Read the model definition and answer for the solid it produces. Units are mm, in the model's axes. Face numbers are marked on the shaded views. A direction names the side the tool comes from. Coordinates: 2 decimals unless noted, no trailing zeros. Order: outer loops, then holes, each group sorted by start corner. A loop starts at its lowest first (then second) coordinate and runs counter-clockwise, first axis right, second up. Notation, with made-up numbers: (80, -3) -> (106, -3) arc R14 ccw to (106, 18) -> close; hole circle Ø8 at (74, 9.5). An arc over 180 degrees is marked (long way). Use CSV: the item, a comma, the result in double quotes.
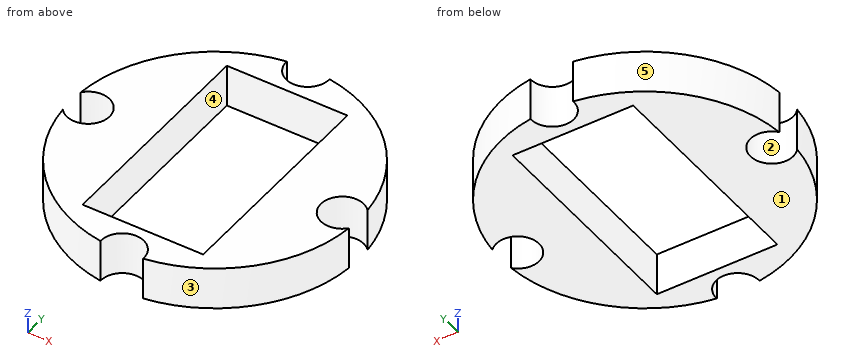
Autodesk Inventor part; units mm, degrees
ref_plane "YZ Plane" through (0, 0, 0) normal (1, 0, 0) x (0, 1, 0)
ref_plane "XZ Plane" through (0, 0, 0) normal (0, 1, 0) x (-1, 0, 0)
ref_plane "XY Plane" through (0, 0, 0) normal (0, 0, 1) x (1, 0, 0)
sketch "Sketch3" plane through (0, 0, 0) normal (0, 0, 1) x (1, 0, 0)
  line L0 (-15.9263, -16.7) -> (16.0737, -16.7)
  line L1 (16.7744, -15.9999) -> (16.6729, 15.9999)
  line L2 (15.9735, 16.7) -> (-16.0265, 16.7)
  line L3 (-16.7272, 15.9999) -> (-16.6257, -15.9999)
  line L4 (-16.0265, 16.7) -> (-16.7272, 15.9999)
  line L5 (15.9735, 16.7) -> (16.6729, 15.9999)
  line L6 (16.7744, -15.9999) -> (16.0737, -16.7)
  line L7 (-16.6257, -15.9999) -> (-15.9263, -16.7)
  line L8 (-5.7625, -10.525) -> (5.7625, -10.525)
  line L9 (5.7625, -10.525) -> (5.7625, 10.525)
  line L10 (5.7625, 10.525) -> (-5.7625, 10.525)
  line L11 (-5.7625, 10.525) -> (-5.7625, -10.525)
  circle A0 centre (-12.159, 13.525) radius 2.045
  circle A1 centre (12.121, 13.525) radius 2.045
  circle A2 centre (-12.0777, -13.525) radius 2.045
  circle A3 centre (12.2023, -13.525) radius 2.045
  circle A4 centre (0, 0) radius 18.4 construction
  circle A5 centre (-12.1163, 0) radius 2.045
  circle A6 centre (0, 13.525) radius 2.045
  circle A7 centre (12.1637, 0) radius 2.045
  circle A8 centre (0, -13.525) radius 2.045
  dimension "d10" = 11.525
  dimension "d11" = 21.05
  dimension "d12" = 4.09
  dimension "d13" = 4.09
  dimension "d17" = 4.09
  dimension "d19" = 24.28
  dimension "d21" = 4.09
  dimension "d26" = 36.8
  dimension "d27" = 4.09
  dimension "d28" = 4.09
  dimension "d29" = 4.09
  dimension "d33" = 4.09
  dimension "d38" = 10.525
  dimension "d39" = 5.7625
  dimension "d45" = 33.4
  dimension "d46" = 33.4
  dimension "d47" = 32
  dimension "d48" = 32
  dimension "d49" = 32
  dimension "d50" = 32
  dimension "d52" = 3
  dimension "d53" = 3
  dimension "d55" = 3
  dimension "d56" = 3
  dimension "d57" = 3
  dimension "d59" = 3
  dimension "d60" = 5.7625
  dimension "d61" = 5.7625
  dimension "d62" = 6.3585
  dimension "d63" = 24.28
  dimension "d64" = 24.28
  dimension "d66" = 10.525
  dimension "d67" = 16.7
sketch "Sketch4" plane through (0, 0, 0) normal (0, 0, 1) x (1, 0, 0)
  circle A0 centre (0, 0) radius 13.75
  dimension "d32" = 27.5
extrude "Extrusion3" add sketch "Sketch3" along normal blind 4.1
extrude "Extrusion4" cut sketch "Sketch4" along normal blind 4.1 keep common part
properties part number "WG18FLANGECutDown"
Item 1: The mould has two halves that part along Y. Classify the marked faces 1, 2 and 3: +Y half, -Y half, draft (parallel to the pull), parting line (faces both ways), or undercut.
Return value:
face 1,"draft"
face 2,"undercut"
face 3,"-Y half"
Item 2: Find section B-B, the plane y = 0. Give the vertices of the cut face in (x, z), then the cut area to 3 significant figures.
Return value:
outline,"(-10.07, 0) -> (-5.76, 0) -> (-5.76, 4.1) -> (-10.07, 4.1) -> close; (5.76, 0) -> (10.12, 0) -> (10.12, 4.1) -> (5.76, 4.1) -> close"
area,"35.5 mm^2"
Item 3: Each of these flat-tipped pins is pushed along its axis until it touches: P1, Ø1.2, axis at x = -3, z = 2, coming from the -Y side; P2, Ø2, axis at y = -9, z = 1, coming from the +X side; P3, Ø2.5, axis at x = 12.16, y = 0, coming from the -Z side; P4, Ø2, axis at y = 0, z = 1.5, coming from the +X side. Where does it stop, or does it pass through?
Return value:
P1,"stops at y = -13.54"
P2,"stops at x = 11.18"
P3,"passes through"
P4,"stops at x = 10.38"
Item 4: Find section A-A, the plane x = 0. Give the vertices of the cut face in (y, z) (3 decimals).
Return value:
outline,"(-11.48, 0) -> (-10.525, 0) -> (-10.525, 4.1) -> (-11.48, 4.1) -> close; (10.525, 0) -> (11.48, 0) -> (11.48, 4.1) -> (10.525, 4.1) -> close"
Item 5: A tool of negligible diameter and unlimited length cuts with its end or side. For the marked faces 4 and 5, from which of +Z, -Z, +X, -X, +Y, -Y can it reach the whole face along a straight path? Write none if from no direction.
Return value:
face 4,"+Z, -Z"
face 5,"+Z, -Z, -X, +Y"
Item 6: Straight lines are drawn through the part: line 1 along X through (y, z) = (5.5, 1.2); line 2 along Y through (x, z) = (11.5, 1.1); line 3 along X through (y, z) = (7, 1.3). For each, find the intervals that lie inside material, in ascending order.
Return value:
line 1,"x = -12.6 to -5.76, 5.76 to 12.6"
line 2,"y = -7.54 to -1.93, 1.93 to 7.54"
line 3,"x = -11.83 to -5.76, 5.76 to 11.83"
